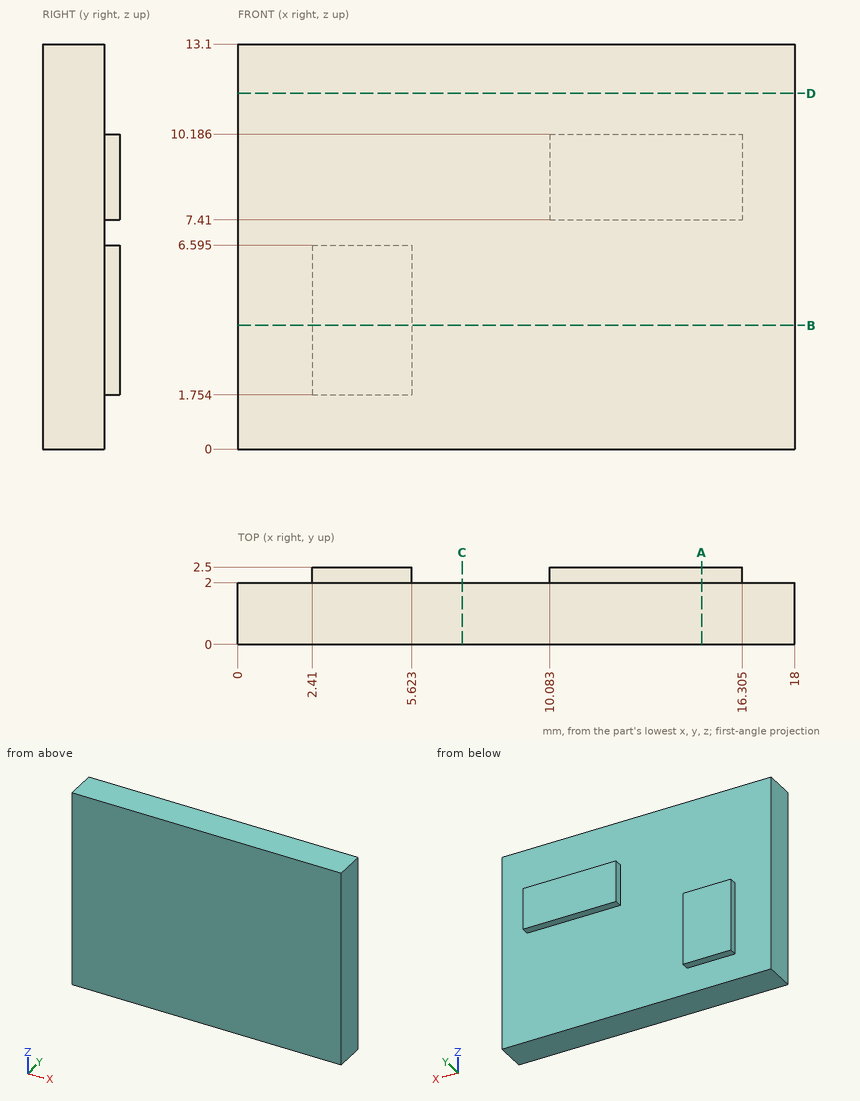
Design review of the part shown in the three views and the two pictorial views. Dimensions are in mm from the part's minimum x, y and z. Round coordinates to 2 decimals unless told otherwise and drop trailing zeros. Write each loop counter-clockwise with the first axis right and the second up, starting at its lowest first coordinate (ties: lowest second). Pieces come first, ordered by that corner, then holes. Notation, with made-up numbers: (60, 28.25) -> (87, 28.25) arc R16 ccw to (87, 51.25) -> close; hole circle Ø7 at (59, 14). An arc over 180 degrees is marked (long way). Answer as a JSON object with one key per item and string values.
1. To check wall thickness, follow line 1 along Y through (x, z) = (8, 12.25); line 2 along Z through (x, y) = (10.75, 2.25) (1 decimal); line 3 along X through (y, z) = (2.2, 3.25). State the ranges of each line that lie inside material, in increasing order.
Results found:
{"line 1": "y = 0 to 2", "line 2": "z = 7.4 to 10.2", "line 3": "x = 2.41 to 5.62"}
2. We need section A-A on x = 15. State the section outline as (y, z) points (1 decimal), and give its area (3 significant figures).
Results found:
{"outline": "(0, 0) -> (2, 0) -> (2, 7.4) -> (2.5, 7.4) -> (2.5, 10.2) -> (2, 10.2) -> (2, 13.1) -> (0, 13.1) -> close", "area": "27.6 mm^2"}
3. We need section D-D on z = 11.5. State the section outline as (x, y) points, and give its area (3 significant figures).
Results found:
{"outline": "(0, 0) -> (18, 0) -> (18, 2) -> (0, 2) -> close", "area": "36.0 mm^2"}
4. We need section B-B on z = 4. State the section outline as (x, y) points.
Results found:
{"outline": "(0, 0) -> (18, 0) -> (18, 2) -> (5.62, 2) -> (5.62, 2.5) -> (2.41, 2.5) -> (2.41, 2) -> (0, 2) -> close"}
5. Clearance check with flat-ended pins moving along their axes: pin 1 (0.6 mm diameter, centred on x = 3, y = 2.5, fed in from -Z); pin 2 (1 mm diameter, centred on x = 7, z = 1.5, fed in from +Y); pin 3 (6 mm diameter, centred on x = 9.5, z = 1.5, fed in from -Y). State where each tip first meets the part, or that it passes through.
Results found:
{"pin 1": "stops at z = 1.75", "pin 2": "stops at y = 2", "pin 3": "stops at y = 0"}
6. We need section C-C on x = 7.25. State the section outline as (y, z) points.
Results found:
{"outline": "(0, 0) -> (2, 0) -> (2, 13.1) -> (0, 13.1) -> close"}
